Verification items for the finished model (mm, model axes). Face numbers are marked on the shaded views. A direction names the side the tool comes from. Round coordinates to 2 decimals unless told otherwise and drop trailing zeros. Order: outer loops, then holes, each group sorted by start corner. A loop starts at its lowest first (then second) coordinate and runs counter-clockwise, first axis right, second up. Notation, with made-up numbers: M 7,7.5 L 58,7.5 A10 cw 58,20.5 Z; hole C 52.5,-39 d7. An arc over 180 degrees is marked long. Use CSV: the item, a comma, the result in double quotes. Start each with the question number.
Q1. Sectioned sample at C-C (z = 4). State how many separate pieces and enclosed holes the cut face has, and give its area (3 significant figures).
Q2. Sectioned sample at A-A (x = 0). Enter the section's corners in (y, z), and give its area (3 significant figures).
Q3. Set-up check for the marked faces 1, 2, 3 and 4: record each of +Z, -Z, +X, -X, +Y, -Y from which the full face is reachable in a straight line by a thin tool's end or side.
Q4. Mould release check, pull along Y, two halves, no side actions. Record for the marked faces 5, 6, 7 and 8: +Y half, -Y half, draft (parallel to the pull), parting line (faces both ways), or undercut.
Q5. Gauge pin test, flat ends, axial feed: pin 1 Ø1 at (x, z) = (58, 27.5) entering from +Y; pin 2 Ø6 at (x, y) = (13.5, 63.5) entering from +Z; pin 3 Ø1.5 at (y, z) = (97.5, 13) entering from +X. Record the tip position at first contact, or that the pin passes through.
Q6. Scan lines: line 1 (X direction, y = 12, z = 6); line 2 (Z direction, x = -66.25, y = 12); line 3 (Y direction, x = -84, z = 40). Record each from-to range of solid material in increasing order.
Q7. Sectioned sample at B-B (y = 69.5). Enter the section's corners in (x, z).
Q8. Sectioned sample at D-D (z = 26). Enter the section's corners in (x, y).
```python
from build123d import *

# Parameters (mm, degrees)
SKETCH1_R           = 4.4
BOSS_EXTRUDE1_DEPTH = 20
FILLET1_R           = 10
SKETCH2_W           = 6.75
SKETCH2_H           = 6.75
CUT_EXTRUDE1_DEPTH  = 124.17331296
SKETCH3_W           = 4.125
SKETCH3_H           = 20
BOSS_EXTRUDE2_DEPTH = 3
FILLET2_R           = 2
BOSS_EXTRUDE3_DEPTH = 20
FILLET3_R           = 10
FILLET4_R           = 2
SKETCH5_R           = 3.1
CUT_EXTRUDE2_DEPTH  = 15
SKETCH6_W           = 185
SKETCH6_H           = 4
BOSS_EXTRUDE4_DEPTH = 42.5
FILLET5_R           = 10
CUT_EXTRUDE3_DEPTH  = 1
SKETCH8_R           = 1.9
CUT_EXTRUDE4_DEPTH  = 10


with BuildPart() as part:
    # Sketch1 → Boss-Extrude1 (new body)
    with BuildSketch(Plane.XY):
        with BuildLine():
            Line((-70, 0), (70, 0))
            Line((70, 0), (70, 12))
            ThreePointArc((70, 12), (66.338834765, 20.838834765), (57.5, 24.5))
            Line((57.5, 24.5), (25, 24.5))
            Line((25, 24.5), (25, 39.5))
            Line((25, 39.5), (44.5, 98.165))
            Line((44.5, 98.165), (29.5, 98.165))
            Line((29.5, 98.165), (0, 9.415384615))
            Line((0, 9.415384615), (-29.5, 98.165))
            Line((-29.5, 98.165), (-44.5, 98.165))
            Line((-44.5, 98.165), (-25, 39.5))
            Line((-25, 39.5), (-25, 24.5))
            Line((-25, 24.5), (-57.5, 24.5))
            ThreePointArc((-57.5, 24.5), (-66.338834765, 20.838834765), (-70, 12))
            Line((-70, 12), (-70, 0))
        make_face()
        with Locations((-57.5, 12)):
            Circle(SKETCH1_R, mode=Mode.SUBTRACT)
        with Locations(Location((57.5, 12, 0), (0, 0, 180))):
            Circle(SKETCH1_R, mode=Mode.SUBTRACT)
    extrude(amount=BOSS_EXTRUDE1_DEPTH)

    # Fillet1
    fillet1_edges = [part.edges().sort_by_distance(p)[0] for p in [
        (25, 39.5, 10),
        (25, 24.5, 10),
        (-25, 24.5, 10),
        (-25, 39.5, 10),
        (0, 9.415384615, 10),
    ]]
    fillet(fillet1_edges, radius=FILLET1_R)

    # Sketch2 → Cut-Extrude1 (cut, through all, along a direction that is not the sketch's normal)
    with BuildSketch(Plane.XY):
        with Locations((37, 98.165)):
            Rectangle(SKETCH2_W, SKETCH2_H)
        with Locations((-37, 98.165)):
            Rectangle(SKETCH2_W, SKETCH2_H)
    extrude(amount=CUT_EXTRUDE1_DEPTH, dir=(0, -0.12403473458920856, 0.9922778767136676), mode=Mode.SUBTRACT)

    # Sketch3 → Boss-Extrude2 (add)
    with BuildSketch(Plane(origin=(0, 98.165, 0), x_dir=(1, 0, 0), z_dir=(0, 1, 0))):
        with Locations((42.4375, -10)):
            Rectangle(SKETCH3_W, SKETCH3_H)
        with Locations((31.5625, -10)):
            Rectangle(SKETCH3_W, SKETCH3_H)
        with Locations((-31.5625, -10)):
            Rectangle(SKETCH3_W, SKETCH3_H)
        with Locations((-42.4375, -10)):
            Rectangle(SKETCH3_W, SKETCH3_H)
    extrude(amount=BOSS_EXTRUDE2_DEPTH)

    # Fillet2
    fillet2_edges = [part.edges().sort_by_distance(p)[0] for p in [
        (-40.375, 93.54, 10),
        (-33.625, 93.54, 10),
        (44.5, 101.165, 10),
        (40.375, 101.165, 10),
        (29.5, 101.165, 10),
        (33.625, 101.165, 10),
        (-29.5, 101.165, 10),
        (-33.625, 101.165, 10),
        (-44.5, 101.165, 10),
        (-40.375, 101.165, 10),
        (44.5, 98.165, 10),
        (33.625, 93.54, 10),
        (40.375, 93.54, 10),
    ]]
    fillet(fillet2_edges, radius=FILLET2_R)

    # Sketch4 → Boss-Extrude3 (add)
    with BuildSketch(Plane.XY.offset(20)):
        Polygon((-22.793222795, 77.98791873), (-7.5, 111.54), (7.5, 111.54), (22.793222795, 77.98791873), (16.196275804, 58.141257439), (0, 93.674563227), (-16.196275804, 58.141257439), align=None)
    extrude(amount=-BOSS_EXTRUDE3_DEPTH)

    # Fillet3
    fillet3_edges = [part.edges().sort_by_distance(p)[0] for p in [
        (0, 93.674563227, 10),
    ]]
    fillet(fillet3_edges, radius=FILLET3_R)

    # Fillet4
    fillet4_edges = [part.edges().sort_by_distance(p)[0] for p in [
        (16.196275804, 58.141257439, 10),
        (22.793222795, 77.98791873, 10),
        (-22.793222795, 77.98791873, 10),
        (-16.196275804, 58.141257439, 10),
    ]]
    fillet(fillet4_edges, radius=FILLET4_R)

    # Sketch5 → Cut-Extrude2 (cut)
    with BuildSketch(Plane(origin=(0, 111.54, 0), x_dir=(1, 0, 0), z_dir=(0, 1, 0))):
        with Locations(Location((0, -10, 0), (0, 0, 270))):
            Circle(SKETCH5_R)
    extrude(amount=-CUT_EXTRUDE2_DEPTH, mode=Mode.SUBTRACT)

    # Sketch6 → Boss-Extrude4 (add)
    with BuildSketch(Plane(origin=(0, 0, 0), x_dir=(-1, 0, 0), z_dir=(0, 0, -1))):
        with Locations((0, 2)):
            Rectangle(SKETCH6_W, SKETCH6_H)
    extrude(amount=-BOSS_EXTRUDE4_DEPTH)

    # Fillet5
    fillet5_edges = [part.edges().sort_by_distance(p)[0] for p in [
        (-92.5, 2, 42.5),
        (92.5, 2, 42.5),
    ]]
    fillet(fillet5_edges, radius=FILLET5_R)

    # Sketch7 → Cut-Extrude3 (cut)
    with BuildSketch(Plane(origin=(0, 24.5, 0), x_dir=(1, 0, 0), z_dir=(0, 1, 0))):
        Polygon((41.25, -9), (46.25, -2), (51.25, -9), (47.75, -9), (47.75, -16), (44.75, -16), (44.75, -9), align=None)
    cut_extrude3 = extrude(amount=-CUT_EXTRUDE3_DEPTH, mode=Mode.SUBTRACT)

    # Sketch8 → Cut-Extrude4 (cut)
    with BuildSketch(Plane(origin=(70, 0, 0), x_dir=(0, 0, -1), z_dir=(1, 0, 0))):
        with Locations((-10, 12)):
            Circle(SKETCH8_R)
    cut_extrude4 = extrude(amount=-CUT_EXTRUDE4_DEPTH, mode=Mode.SUBTRACT)

    # Mirror1: Cut-Extrude3, Cut-Extrude4 across plane
    add(cut_extrude3.mirror(Plane(origin=(0, 0, 0), x_dir=(0, 0, 1), z_dir=(1, 0, 0))), mode=Mode.SUBTRACT)
    add(cut_extrude4.mirror(Plane(origin=(0, 0, 0), x_dir=(0, 0, 1), z_dir=(1, 0, 0))), mode=Mode.SUBTRACT)


solid = part.part
```
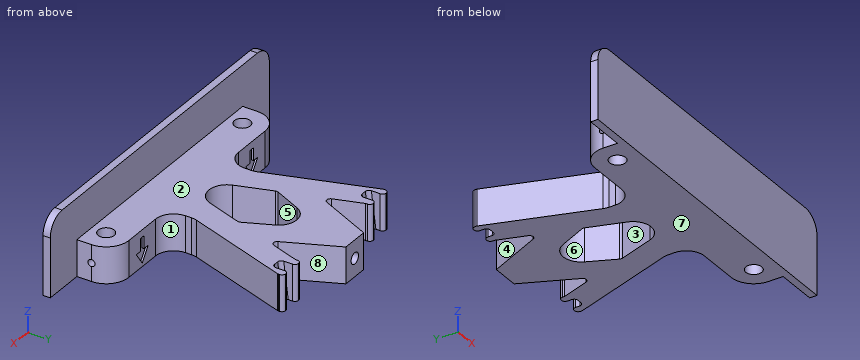
Verdict:
1,separate pieces,"1"
1,enclosed holes,"3"
1,area,"7,170 mm²"
2,outline,"M 0,0 L 31.12,0 L 31.12,20 L 4,20 L 4,42.5 L 0,42.5 Z; M 79.56,0 L 111.54,0 L 111.54,6.9 L 96.54,6.9 L 96.54,13.1 L 111.54,13.1 L 111.54,20 L 79.56,20 Z"
2,area,"1,260 mm²"
3,face 1,"+Z, -Z, +X"
3,face 2,"+Z, +X, -X, +Y"
3,face 3,"+Z, -Z"
3,face 4,"+Z, -Z, +Y"
4,face 5,"undercut"
4,face 6,"undercut"
4,face 7,"draft"
4,face 8,"+Y half"
5,pin 1,"stops at y = 4"
5,pin 2,"stops at z = 20"
5,pin 3,"stops at x = 44.49"
6,line 1,"x = -70 to -61.9, -53.1 to 53.1, 61.9 to 70"
6,line 2,"z = 0 to 8.1, 11.9 to 20"
6,line 3,"y = 0 to 4"
7,outline,"M -34.97,0 L -11.02,0 L -11.02,20 L -34.97,20 Z; M 11.02,0 L 34.97,0 L 34.97,20 L 11.02,20 Z"
8,outline,"M -92.5,0 L 92.5,0 L 92.5,4 L -92.5,4 Z"
